Model file for the job. Use its own axes, mm. A direction names the side the tool comes from. Coordinates: 2 decimals unless noted, no trailing zeros. Loops run counter-clockwise (first coordinate to the right, second up) from the corner with the lowest first, then second, coordinate; pieces in that order, holes last. Notation, with made-up numbers: (69, 30) - (110, 30) arc R14 ccw to (110, 46) - close; hole circle Ø3 at (70, 12). An arc over 180 degrees is marked (long way). Write each question's results on one line, items separated by ' | '. Start each with the question number.
```python
from build123d import *

# Parameters (mm, degrees)
SKETCH1_R           = 85
BOSS_EXTRUDE2_DEPTH = 10
SKETCH3_W           = 30
SKETCH3_H           = 81
SKETCH3_W_2         = 60
SKETCH3_H_2         = 40
SKETCH3_W_3         = 65
SKETCH3_H_3         = 70
CUT_EXTRUDE2_DEPTH  = 7
SKETCH5_W           = 194.063046405
SKETCH5_H           = 184.49419377
CUT_EXTRUDE4_DEPTH  = 10
BOSS_EXTRUDE3_DEPTH = 20


with BuildPart() as part:
    # Sketch1 → Boss-Extrude2 (new body)
    with BuildSketch(Plane(origin=(0, 0, 0), x_dir=(1, 0, 0), z_dir=(0, 1, 0))):
        Circle(SKETCH1_R)
    extrude(amount=BOSS_EXTRUDE2_DEPTH)

    # Sketch3 → Cut-Extrude2 (cut)
    with BuildSketch(Plane(origin=(0, 10, 0), x_dir=(1, 0, 0), z_dir=(0, 1, 0))):
        with Locations((-50, 0)):
            Rectangle(SKETCH3_W, SKETCH3_H)
        with Locations((10, 45)):
            Rectangle(SKETCH3_W_2, SKETCH3_H_2)
        with Locations((7.5, -30)):
            Rectangle(SKETCH3_W_3, SKETCH3_H_3)
    extrude(amount=-CUT_EXTRUDE2_DEPTH, mode=Mode.SUBTRACT)

    # Sketch5 → Cut-Extrude4 (cut)
    with BuildSketch(Plane(origin=(0, 10, 0), x_dir=(1, 0, 0), z_dir=(0, 1, 0))):
        with Locations((-1.510871468, -0.083937304)):
            Rectangle(SKETCH5_W, SKETCH5_H)
        Polygon((-70, 43), (-20, 72.5), (40, 72.5), (69.5, 22.5), (69.5, -22.5), (40, -72.5), (-25, -72.5), (-70, -43), align=None, mode=Mode.SUBTRACT)
    extrude(amount=-CUT_EXTRUDE4_DEPTH, mode=Mode.SUBTRACT)

    # Sketch6 → Boss-Extrude3 (add)
    with BuildSketch(Plane(origin=(0, 10, 0), x_dir=(1, 0, 0), z_dir=(0, 1, 0))):
        Polygon((-70, 43), (-20, 72.5), (38.257502672, 72.5), (40, 72.5), (69.5, 22.5), (69.5, -22.5), (40, -72.5), (-25, -72.5), (-70, -43), align=None)
        Polygon((-65, 40.5), (-65, -40.5), (-25, -65), (40, -65), (64.618640633, -22.5), (64.618640633, 22.5), (40, 65), (-20, 65), align=None, mode=Mode.SUBTRACT)
    extrude(amount=BOSS_EXTRUDE3_DEPTH)


solid = part.part
```
Q1. Cut at D-D (x = -15.5). List the corners of the cut face in (y, z).
Q2. Which spindle directions (+Z, -Z, +X, -X, +Y, -Y) get a long thin tool onto all of the face, cutting with end or side? Do faces 4 (the flat face through (-20, 7, -45)), 5 (the flat face through (-70, 15, 1)). Say none if no direction does.
Q3. Cut at C-C (y = 21.25). List the corners of the cut face in (x, z).
Q4. Cut at A-A (y = 7). List the corners of the cut face in (x, z).
Q5. Pin check, flat tips, straight feed: pin 1 (3.5 mm diameter, centred on x = -55.5, y = 6.5, fed in from +Z); pin 2 (5.5 mm diameter, centred on y = 8, z = -39.5, fed in from +X); pin 3 (4 mm diameter, centred on x = -27.5, z = -25, fed in from -Y); pin 4 (2 mm diameter, centred on x = -43, y = 7.5, fed in from -Z). Stop position of each tip, or through.
Q6. Cut at B-B (z = 12). List the corners of the cut face in (x, y).
Q7. Mould opens along X. For faces 1 (the flat face through (54.544, 14.79, -47.85)), 2 (the flat face through (-67, 30, 0)), 3 (the flat face through (-65, 16, -1)) say: +X half, -X half, draft (parallel to the pull), parting line (faces both ways), or undercut.
Q8. Drill centre lines: L1, parallel to X at y = 8, z = 1; L2, parallel to X at y = 9.5, z = -35 (3 decimals); L3, parallel to Z at x = 10, y = 13.25. Where is each one in solid material? Low to high. Write a range as from..to.
Check result:
1) outline: (0, -72.5) - (30, -72.5) - (30, -65) - (3, -65) - (3, -25) - (10, -25) - (10, -5) - (3, -5) - (3, 65) - (30, 65) - (30, 72.5) - (0, 72.5) - close
2) face 4: +Y | face 5: +Z, -Z, -X, +Y, -Y
3) outline: (-70, -43) - (-20, -72.5) - (40, -72.5) - (69.5, -22.5) - (69.5, 22.5) - (40, 72.5) - (-25, 72.5) - (-70, 43) - close; hole (-65, -40.5) - (-20, -65) - (40, -65) - (64.62, -22.5) - (64.62, 22.5) - (40, 65) - (-25, 65) - (-65, 40.5) - close
4) outline: (-70, -43) - (-20, -72.5) - (40, -72.5) - (69.5, -22.5) - (69.5, 22.5) - (40, 72.5) - (-25, 72.5) - (-70, 43) - close; hole (-65, -40.5) - (-35, -40.5) - (-35, 40.5) - (-65, 40.5) - close; hole (-25, -5) - (40, -5) - (40, 65) - (-25, 65) - close; hole (-20, -65) - (40, -65) - (40, -25) - (-20, -25) - close
5) pin 1: z = 53.65 | pin 2: x = 61.09 | pin 3: y = 0 | pin 4: z = -59.52
6) outline: (-70, 0) - (69.5, 0) - (69.5, 30) - (64.62, 30) - (64.62, 10) - (40, 10) - (40, 3) - (-25, 3) - (-25, 10) - (-35, 10) - (-35, 3) - (-65, 3) - (-65, 30) - (-70, 30) - close
7) face 1: +X half | face 2: draft | face 3: undercut
8) L1: -70..-65, -35..-25, 40..69.5 | L2: -70..-65, -35..-20, 40..62.125 | L3: -72.5..-65, 65..72.5
